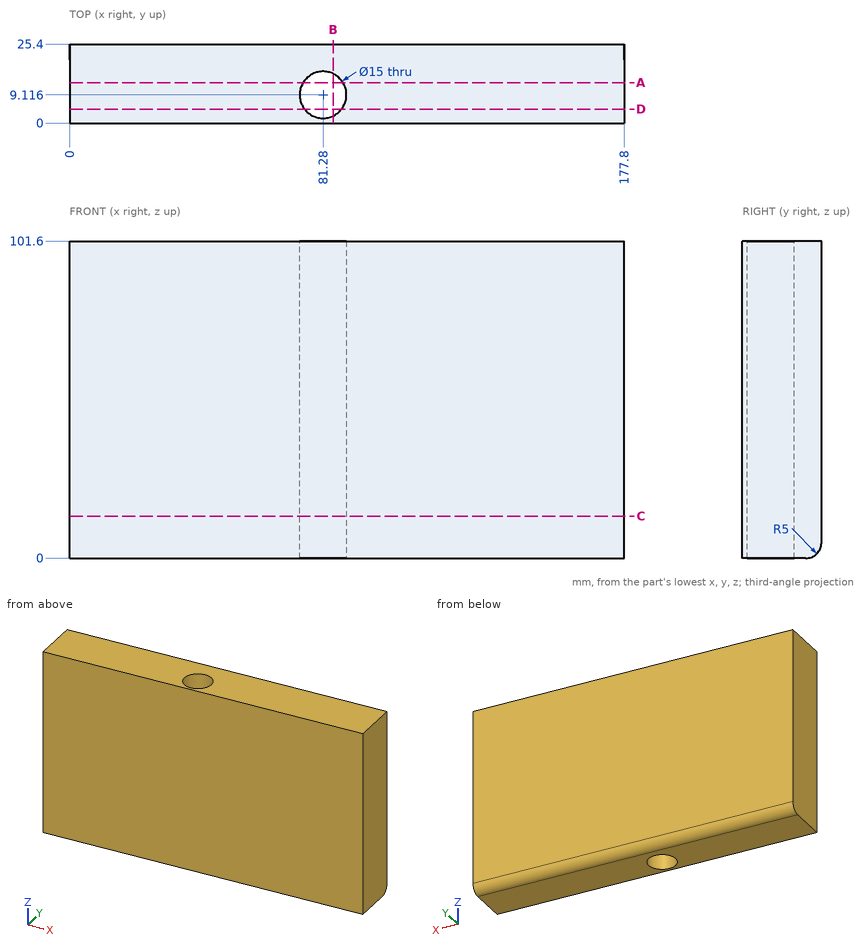
Geometry: see drawing. Coordinates: mm, zero at the bounding-box minimum. Round coordinates to 2 decimals unless told otherwise and drop trailing zeros. Loops run counter-clockwise (first coordinate to the right, second up) from the corner with the lowest first, then second, coordinate; pieces in that order, holes last. Notation, with made-up numbers: (36.5, -29) -> (56.5, -29) arc R20 cw to (56.5, -8) -> close; hole circle Ø1 at (1.5, 68). An arc over 180 degrees is marked (long way). One line per question, with ' | ' between items. Start each with the question number.
1. Section A-A on y = 13. Output: boundary loops of the cut face in (x, z) (1 decimal), and give its area (3 significant figures).
2. Section C-C on z = 13.5. Output: boundary loops of the cut face in (x, y), and give its area (3 significant figures).
3. Section D-D on y = 4.5. Output: boundary loops of the cut face in (x, z).
4. Section B-B on x = 84.5. Output: boundary loops of the cut face in (y, z), and give its area (3 significant figures).
5. Line query: line 1 along X through (y, z) = (13, 16) (1 decimal); line 2 along X through (y, z) = (3, 20.5); line 3 along Z through (x, y) = (118.5, 21.75) (1 decimal). Output: solid intervals per line, ascending. Write a range as [from, to].
Returned:
1) outline: (0, 0) -> (74.9, 0) -> (74.9, 101.6) -> (0, 101.6) -> close; (87.7, 0) -> (177.8, 0) -> (177.8, 101.6) -> (87.7, 101.6) -> close | area: 16,800 mm2
2) outline: (0, 0) -> (177.8, 0) -> (177.8, 25.4) -> (0, 25.4) -> close; hole circle Ø15 at (81.28, 9.12) | area: 4,340 mm2
3) outline: (0, 0) -> (75.37, 0) -> (75.37, 101.6) -> (0, 101.6) -> close; (87.19, 0) -> (177.8, 0) -> (177.8, 101.6) -> (87.19, 101.6) -> close
4) outline: (0, 0) -> (2.34, 0) -> (2.34, 101.6) -> (0, 101.6) -> close; (15.89, 0) -> (20.4, 0) arc R5 ccw to (25.4, 5) -> (25.4, 101.6) -> (15.89, 101.6) -> close | area: 1,200 mm2
5) line 1: x = [0, 74.9], [87.7, 177.8] | line 2: x = [0, 76.94], [85.62, 177.8] | line 3: z = [0.2, 101.6]
